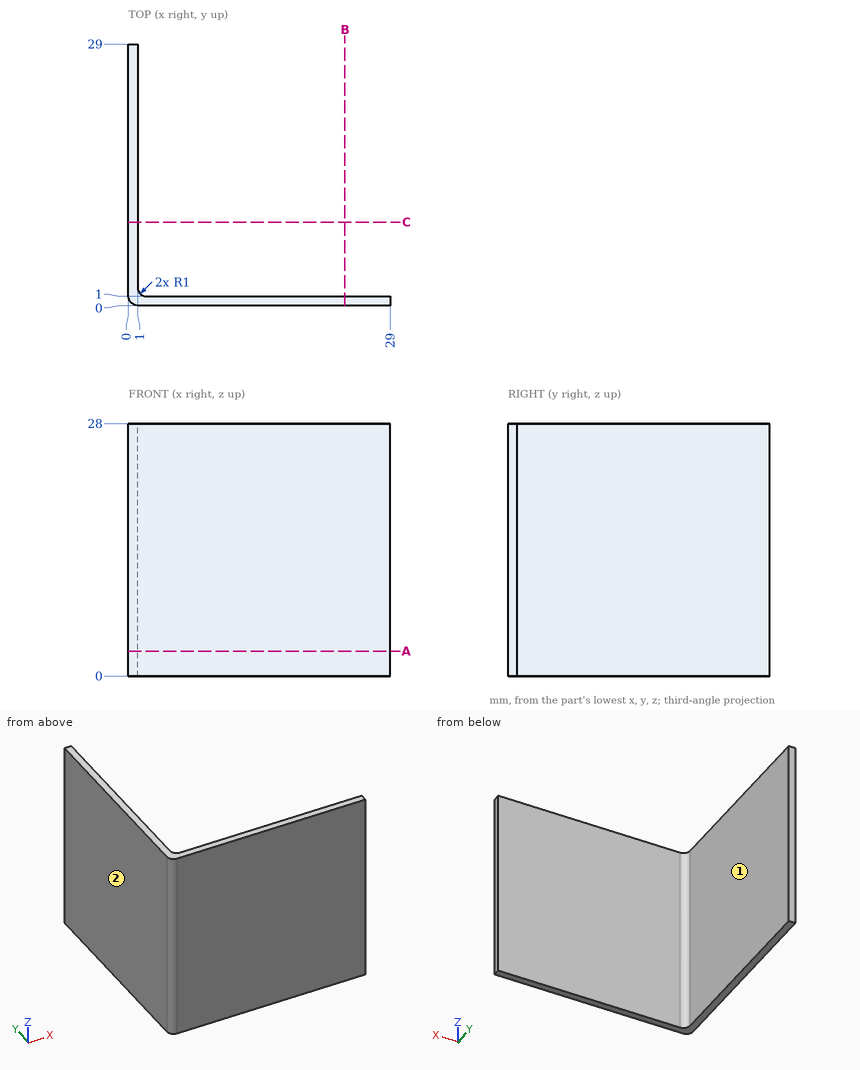
Geometry check sheet. Reference: drawing and pictorial views, mm from the part's lowest x, y, z. A direction names the side the tool comes from. Round coordinates to 2 decimals unless told otherwise and drop trailing zeros. Loops run counter-clockwise (first coordinate to the right, second up) from the corner with the lowest first, then second, coordinate; pieces in that order, holes last. Notation, with made-up numbers: (86.25, 45.25) - (103.25, 45.25) arc R12 cw to (103.25, 50.25) - close; hole circle Ø4 at (71.25, -15.5). An arc over 180 degrees is marked (long way). Answer as CSV lines item,"result".
(1) Set-up check for the marked faces 1 and 2: record each of +Z, -Z, +X, -X, +Y, -Y from which the full face is reachable in a straight line by a thin tool's end or side.
Output values:
face 1,"+Z, -Z, +X, +Y"
face 2,"+Z, -Z, -X, +Y, -Y"
(2) Depth check by flat-ended pin: pin 1 Ø6 at (x, z) = (12.5, 19.5) entering from +Y; pin 2 Ø3 at (y, z) = (18, 10.5) entering from +X. Enter the tip coordinate at first touch or a pass-through.
Output values:
pin 1,"stops at y = 1"
pin 2,"stops at x = 1"
(3) Material ranges on line 1 along Y through (x, z) = (5.25, 18.25), recorded low to high.
Output values:
line 1,"y = 0 to 1"
(4) Cross-section at B-B, the plane x = 24. Enter the section's corners in (y, z), and give its area (3 significant figures).
Output values:
outline,"(0, 0) - (1, 0) - (1, 28) - (0, 28) - close"
area,"28.0 mm²"
(5) Cross-section at A-A, the plane z = 2.75. Enter the section's corners in (x, y).
Output values:
outline,"(0, 1) arc R1 ccw to (1, 0) - (29, 0) - (29, 1) - (2, 1) arc R1 cw to (1, 2) - (1, 29) - (0, 29) - close"
